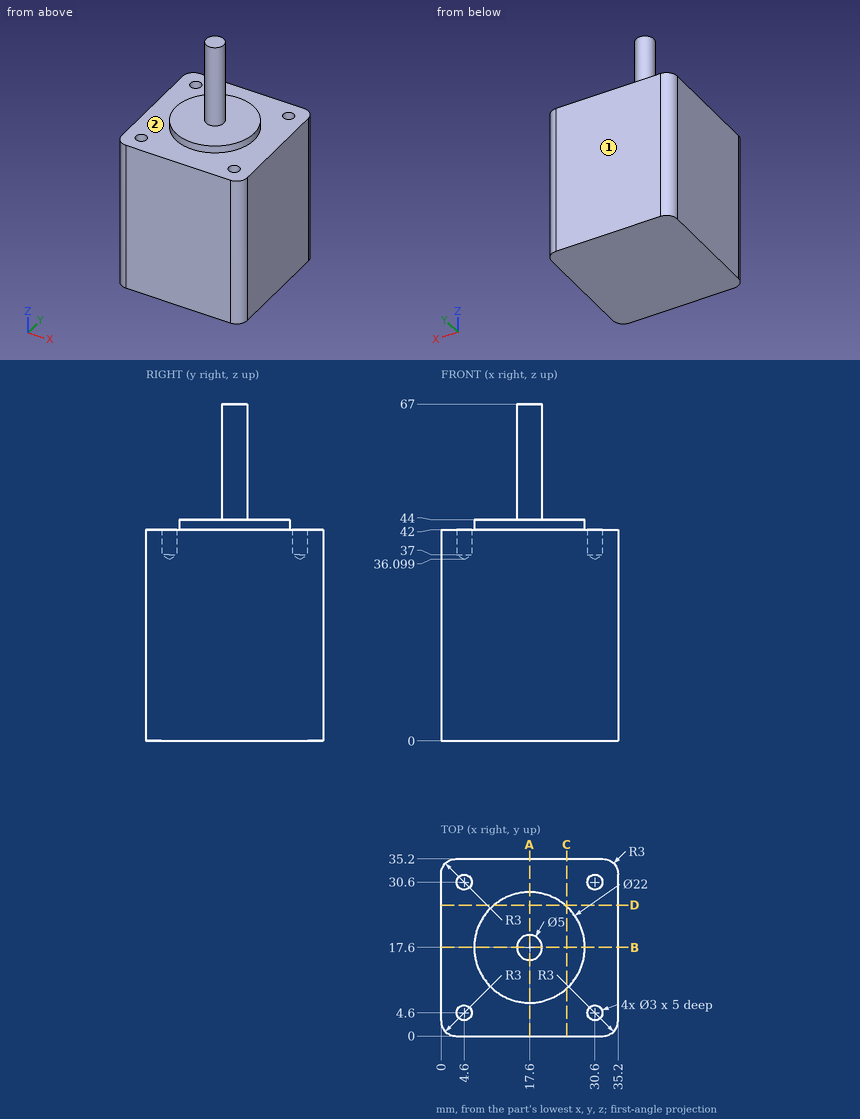
For this review, use the dimensioned drawing (mm, ordinates from the lowest corner) and the shaded views. A direction names the side the tool comes from. Round coordinates to 2 decimals unless told otherwise and drop trailing zeros. Write each loop counter-clockwise with the first axis right and the second up, starting at its lowest first coordinate (ties: lowest second). Pieces come first, ordered by that corner, then holes. Notation, with made-up numbers: (-1.5, 44) -> (3.5, 44) arc R27 cw to (3.5, 74) -> close; hole circle Ø2 at (17.25, -17). An arc over 180 degrees is marked (long way). Use CSV: the item, a comma, the result in double quotes.
Q1. For pin 1 Ø6 at (x, z) = (16, 50.5) entering from -Y; pin 2 Ø2.5 at (x, y) = (30.6, 30.6) entering from +Z, all flat-tipped, find the tip position at first contact; note any pin that passes through.
Checks:
pin 1,"y = 15.1"
pin 2,"z = 36.85"
Q2. Consider section C-C (x = 25). Give the boundary of the cut face in (y, z).
Checks:
outline,"(0, 0) -> (35.2, 0) -> (35.2, 42) -> (25.74, 42) -> (25.74, 44) -> (9.46, 44) -> (9.46, 42) -> (0, 42) -> close"
Q3. Consider section A-A (x = 17.6). Give the boundary of the cut face in (y, z), then the cut area to 3 significant figures.
Checks:
outline,"(0, 0) -> (35.2, 0) -> (35.2, 42) -> (28.6, 42) -> (28.6, 44) -> (20.1, 44) -> (20.1, 67) -> (15.1, 67) -> (15.1, 44) -> (6.6, 44) -> (6.6, 42) -> (0, 42) -> close"
area,"1,640 mm²"
Q4. For the marked faces 1 and 2, list the 3-axis set-ups (+Z, -Z, +X, -X, +Y, -Y) from which the entire face can be reached by the end or side of a thin tool; tool diameter is ignored.
Checks:
face 1,"+Z, -Z, +X, -X, +Y"
face 2,"+Z"
Q5. To check wall thickness, follow probe 1 along Y at (x, z) = (30.6, 38.8); probe 2 along X at (y, z) = (30, 39) (1 decimal). State the ranges of each line that lie inside material, in increasing order. Write a range as [from, to].
Checks:
probe 1,"[0, 3.1], [6.1, 29.1], [32.1, 35.2]"
probe 2,"[0, 3.2], [6, 29.2], [32, 35.2]"
Q6. Consider section D-D (y = 26). Give the boundary of the cut face in (x, z).
Checks:
outline,"(0, 0) -> (35.2, 0) -> (35.2, 42) -> (24.7, 42) -> (24.7, 44) -> (10.5, 44) -> (10.5, 42) -> (0, 42) -> close"
